Can you work these out from the model? Positions are in its coordinate system, mm. A direction names the side the tool comes from. Give positions to 0.01 mm unless a question says otherwise; leave off trailing zeros. Order: outer loops, then holes, each group sorted by start corner. A loop starts at its lowest first (then second) coordinate and runs counter-clockwise, first axis right, second up. Notation, with made-up numbers: (-11, 71) -> (17, 71) arc R33 ccw to (17, 105) -> close; hole circle Ø8 at (-26, 35). An arc over 180 degrees is marked (long way). Answer as CSV lines item,"result".
```python
from build123d import *

# Parameters (mm, degrees)
PAD_DEPTH    = 0.8
SKETCH001_R  = 20
PAD001_DEPTH = 4
SKETCH002_R  = 19
POCKET_DEPTH = 4.801


with BuildPart() as part:
    # Sketch → Pad (new body)
    with BuildSketch(Plane.XY):
        with BuildLine():
            ThreePointArc((0, 20), (-14.142136, 14.142136), (-20, 0))
            Line((-27, 0), (-20, 0))
            ThreePointArc((-27, 0), (-19.091883, -19.091883), (0, -27))
            Line((0, -27), (0, -20))
            ThreePointArc((0, -20), (14.142136, -14.142136), (20, 0))
            Line((27, 0), (20, 0))
            ThreePointArc((27, 0), (19.091883, 19.091883), (0, 27))
            Line((0, 27), (0, 20))
        make_face()
    extrude(amount=PAD_DEPTH)

    # Sketch001 → Pad001 (new body)
    with BuildSketch(Plane.XY.offset(0.8)):
        Circle(SKETCH001_R)
    extrude(amount=PAD001_DEPTH)

    # Sketch002 → Pocket (cut, through all)
    with BuildSketch(Plane.XY.offset(4.8)):
        Circle(SKETCH002_R)
    extrude(amount=-POCKET_DEPTH, mode=Mode.SUBTRACT)


solid = part.part
```
Item 1: For faces 4 (the flat face through (8, -18, 0)), 5 (the flat face through (15, 15, 0.8)), which set-ups out of +Z, -Z, +X, -X, +Y, -Y let a thin tool reach every point of the face, with its end or its side?
Numbers:
face 4,"-Z, +X, -X, +Y, -Y"
face 5,"+Z, +X, +Y"
Item 2: For pin 1 (2 mm diameter, centred on x = -5, z = 4, fed in from -Y); pin 2 (8 mm diameter, centred on x = 7, y = -14.5, fed in from -Z); pin 3 (23 mm diameter, centred on x = 0, y = 0, fed in from +Z); pin 4 (0.6 mm diameter, centred on x = 23, z = 0, fed in from -Y), each with a flat end and sliding along its axis, tell me the tip position at first contact or that it passes through.
Numbers:
pin 1,"stops at y = -19.6"
pin 2,"stops at z = 0"
pin 3,"passes through"
pin 4,"stops at y = 0"
Item 3: Imagine slicing it at A-A, the plane y = -14. Please give me the cut outline in (x, z), then the cut area to 3 significant figures.
Numbers:
outline,"(-23.09, 0) -> (-12.85, 0) -> (-12.85, 4.8) -> (-14.28, 4.8) -> (-14.28, 0.8) -> (-23.09, 0.8) -> close; (12.85, 0) -> (14.28, 0) -> (14.28, 4.8) -> (12.85, 4.8) -> close"
area,"20.8 mm²"
Item 4: Imagine slicing it at D-D, the plane y = -22.5. Please give me the cut outline in (x, z), then the cut area to 3 significant figures.
Numbers:
outline,"(-14.92, 0) -> (0, 0) -> (0, 0.8) -> (-14.92, 0.8) -> close"
area,"11.9 mm²"
Item 5: Please list where these lines run through material, in increasing order: line 1 along Y through (x, z) = (0, 1.9); line 2 along X through (y, z) = (13, 1.6); line 3 along Y through (x, z) = (-13.5, 3.35).
Numbers:
line 1,"y = -20 to -19, 19 to 20"
line 2,"x = -15.2 to -13.86, 13.86 to 15.2"
line 3,"y = -14.76 to -13.37, 13.37 to 14.76"
Item 6: We'd pull the mould along X, two halves only. Please class faces 1 (the flat face through (-15, -15, 0.8)), 2 (the cylindrical face through (8.767, -16.856, 2.434)), 3 (the cylindrical face through (-19.3, -18.88, 0.39)): released by +X, released by -X, zero draft, split by the parting line, or undercut.
Numbers:
face 1,"zero draft"
face 2,"undercut"
face 3,"released by -X"
Item 7: Imagine slicing it at B-B, the plane x = 16. Please give me the cut outline in (y, z).
Numbers:
outline,"(-12, 0) -> (-10.25, 0) -> (-10.25, 4.8) -> (-12, 4.8) -> close; (10.25, 0) -> (21.75, 0) -> (21.75, 0.8) -> (12, 0.8) -> (12, 4.8) -> (10.25, 4.8) -> close"
Item 8: Imagine slicing it at C-C, the plane z = 3.6. Please give me the cut outline in (x, y), then the cut area to 3 significant figures.
Numbers:
outline,"circle Ø40 at (0, 0); hole circle Ø38 at (0, 0)"
area,"123 mm²"
